```python
from build123d import *

# Parameters (mm, degrees)
SKETCH1_R           = 9.5
SKETCH1_R_2         = 1.5494
BOSS_EXTRUDE1_DEPTH = 3.175


# Read off the part's stored shape, not the designer's step: Imported1
with BuildPart() as part:
    # Sketch1 → Boss-Extrude1 (new body)
    with BuildSketch(Plane(origin=(2.25, 0, 0), x_dir=(0, 0, -1), z_dir=(1, 0, 0))):
        with Locations(Location((0, 0, 0), (0, 0, 90))):
            Circle(SKETCH1_R)
        with Locations(Location((-6.35, 0, 0), (0, 0, 90))):
            Circle(SKETCH1_R_2, mode=Mode.SUBTRACT)
        with Locations(Location((6.35, 0, 0), (0, 0, 90))):
            Circle(SKETCH1_R_2, mode=Mode.SUBTRACT)
        with BuildLine():
            Line((-1.024695077, 1.6), (1.024695077, 1.6))
            ThreePointArc((1.024695077, 1.6), (0, -1.9), (-1.024695077, 1.6))
        make_face(mode=Mode.SUBTRACT)
    extrude(amount=BOSS_EXTRUDE1_DEPTH)


solid = part.part
```
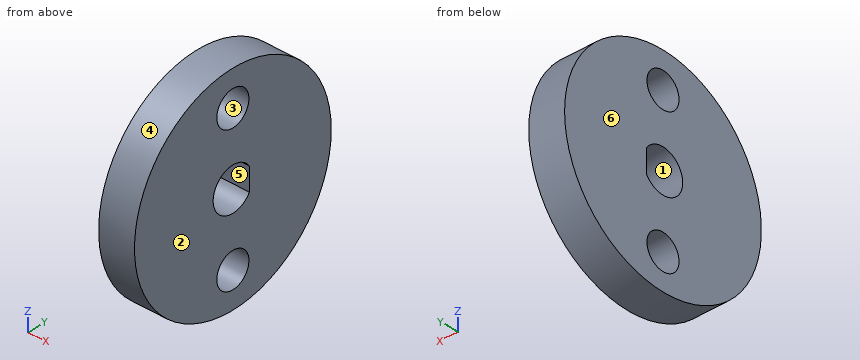
Geometry: final body of the model. Coordinates: model frame, mm. Face numbers are marked on the shaded views. A direction names the side the tool comes from. Give positions to 0.01 mm unless a question says otherwise; leave off trailing zeros. Loops run counter-clockwise (first coordinate to the right, second up) from the corner with the lowest first, then second, coordinate; pieces in that order, holes last. Notation, with made-up numbers: (-20, -12.75) -> (-3, -12.75) arc R29 cw to (-3, 22.25) -> close; hole circle Ø3 at (-12, 46). An arc over 180 degrees is marked (long way). Use CSV: the item, a comma, the result in double quotes.
(1) Cut plane A-A (y = 0). Output: boundary loops of the cut face in (x, z) (3 decimals), plus the area to 3 significant figures.
From the geometry:
outline,"(2.25, -9.5) -> (5.425, -9.5) -> (5.425, -7.899) -> (2.25, -7.899) -> close; (2.25, -4.801) -> (5.425, -4.801) -> (5.425, -1.9) -> (2.25, -1.9) -> close; (2.25, 1.9) -> (5.425, 1.9) -> (5.425, 4.801) -> (2.25, 4.801) -> close; (2.25, 7.899) -> (5.425, 7.899) -> (5.425, 9.5) -> (2.25, 9.5) -> close"
area,"28.6 mm^2"
(2) Cut plane B-B (z = 0). Output: boundary loops of the cut face in (x, y) (3 decimals), plus the area to 3 significant figures.
From the geometry:
outline,"(2.25, -9.5) -> (5.425, -9.5) -> (5.425, -1.9) -> (2.25, -1.9) -> close; (2.25, 1.6) -> (5.425, 1.6) -> (5.425, 9.5) -> (2.25, 9.5) -> close"
area,"49.2 mm^2"
(3) Access query for the marked faces 5 and 6. Directions: +Z, -Z, +X, -X, +Y, -Y. A direction counts if a zero-diameter tool reaches every point of the face in a straight line with its end or side. Return the directions, or none.
From the geometry:
face 5,"+X, -X"
face 6,"+Z, -Z, -X, +Y, -Y"
(4) Ray query, line 1 along Z through (x, y) = (3.1, 0); line 2 along Y through (x, z) = (2.85, 1); line 3 along Y through (x, z) = (4.1, -5.25). Return the intervals inside material, ascending. Write a range as [from, to].
From the geometry:
line 1,"[-9.5, -7.9], [-4.8, -1.9], [1.9, 4.8], [7.9, 9.5]"
line 2,"[-9.45, -1.62], [1.6, 9.45]"
line 3,"[-7.92, -1.09], [1.09, 7.92]"
(5) Cut plane D-D (z = -6.35). Output: boundary loops of the cut face in (x, y) (3 decimals), plus the area to 3 significant figures.
From the geometry:
outline,"(2.25, -7.066) -> (5.425, -7.066) -> (5.425, -1.549) -> (2.25, -1.549) -> close; (2.25, 1.549) -> (5.425, 1.549) -> (5.425, 7.066) -> (2.25, 7.066) -> close"
area,"35.0 mm^2"
(6) First-contact query: P1, Ø1.9, axis at y = 0, z = 6.35, coming from the +X side; P2, Ø0.6, axis at x = 3.5, z = -0.5, coming from the -Y side; P3, Ø5, axis at y = 0, z = 0, coming from the -X side. Flat tips, straight axial feed; report the tip coordinate or a pass-through.
From the geometry:
P1,"through"
P2,"y = -9.5"
P3,"x = 2.25"
(7) Pull-direction query (Z, two-part tool) for the marked faces 1, 2, 3 and 4; classes: released by +Z, released by -Z, zero draft, split by the parting line, or undercut.
From the geometry:
face 1,"undercut"
face 2,"zero draft"
face 3,"undercut"
face 4,"split by the parting line"
(8) Cut plane C-C (x = 4.85). Output: boundary loops of the cut face in (y, z).
From the geometry:
outline,"circle Ø19 at (0, 0); hole circle Ø3.1 at (0, -6.35); hole circle Ø3.1 at (0, 6.35); hole (1.6, -1.02) -> (1.6, 1.02) arc R1.9 ccw (long way) to start"
